Could you check a few things on this model? Use its own coordinates, in mm. A direction names the side the tool comes from. Give positions to 0.01 mm unless a question says otherwise; leave off trailing zeros. Order: outer loops, then holes, each group sorted by start corner. A loop starts at its lowest first (then second) coordinate and runs counter-clockwise, first axis right, second up. Notation, with made-up numbers: M -40,-39 L -16,-39 A35 cw -16,-5 Z; hole C 19,40.25 d8. An arc over 180 degrees is marked long. Use a Markdown table: item, result. Add a question column.
Autodesk Inventor part; units mm, degrees
ref_plane "YZ Plane" through (0, 0, 0) normal (1, 0, 0) x (0, 1, 0)
ref_plane "XZ Plane" through (0, 0, 0) normal (0, 1, 0) x (-1, 0, 0)
ref_plane "XY Plane" through (0, 0, 0) normal (0, 0, 1) x (1, 0, 0)
sketch "Skizze1" plane through (0, 0, 0) normal (0, 0, 1) x (1, 0, 0)
  line L0 (-21, 21) -> (21, 21)
  line L1 (21, 21) -> (21, -21)
  line L2 (21, -21) -> (-21, -21)
  line L3 (-21, -21) -> (-21, 21)
  line L4 (-29.4, 0) -> (29.4, 0)
  line L5 (0, -29.4) -> (0, 29.4)
  point P0 (0, 0)
  dimension "d0" = 42
  dimension "d1" = 42
extrude "Extrusion1" add sketch "Skizze1" along normal blind 50
sketch "Skizze2" plane through (0, 0, 50) normal (0, 0, 1) x (1, 0, 0)
  circle A0 centre (0, 0) radius 11
  dimension "d4" = 22
extrude "Extrusion2" add sketch "Skizze2" along normal blind 2
sketch "Skizze3" plane through (0, 0, 52) normal (0, 0, 1) x (1, 0, 0)
  circle A0 centre (0, 0) radius 11
  circle A1 centre (0, 0) radius 2.5
  dimension "d7" = 5
extrude "Extrusion3" add sketch "Skizze3" along normal blind 22 contours A1
chamfer "Fase1" distance 5 angle 45 4 edges at (-21, -21, 25) (21, -21, 25) (21, 21, 25) (-21, 21, 25)
sketch "Skizze4" plane through (0, 0, 50) normal (0, 0, 1) x (1, 0, 0)
  line L0 (-15.5, 15.5) -> (15.5, 15.5)
  line L1 (15.5, 15.5) -> (15.5, -15.5)
  line L2 (15.5, -15.5) -> (-15.5, -15.5)
  line L3 (-15.5, -15.5) -> (-15.5, 15.5)
  line L4 (-29.4, 0) -> (29.4, 0)
  line L5 (0, -29.4) -> (0, 29.4)
  dimension "d13" = 31
hole "Bohrung1" at (-15.5, 15.5, 50) at (15.5, 15.5, 50) at (15.5, -15.5, 50) at (-15.5, -15.5, 50) direction (0, 0, -1) diameter 2.459 depth 4.5 tip angle 118
properties part number "Motor"
1) Suppose I cut it at A-A on z = 5. Please give me the cut outline in (x, y).
2) For faces 4 (the face through (21, 0, 25)), 5 (the face through (-0.54, 2.44, 62.85)), which set-ups out of +Z, -Z, +X, -X, +Y, -Y let a thin tool reach every point of the face, with its end or its side?
3) For pin 1 (1.5 mm diameter, centred on x = 15.5, y = 15.5, fed in from +Z); pin 2 (4 mm diameter, centred on x = 7, z = 53, fed in from +Y); pin 3 (12.5 mm diameter, centred on x = 8.5, y = 4.5, fed in from +Z), each with a flat end and sliding along its axis, tell me the tip position at first contact or that it passes through.
4) Suppose I cut it at B-B on y = 0. Please give me the cut outline in (x, z), and give its area (3 significant figures).
5) We'd pull the mould along Y, two halves only. Please class faces 1 (the face through (0, 0, 74)), 2 (the face through (-18, -19, 25)), 3 (the face through (-15.869, -16.673, 47.718)): pulls with the +Y half, pulls with the -Y half, needs draft (parallel to the pull), parting line crosses it, or undercut.
6) Suppose I cut it at D-D on y = 18. Please give me the cut outline in (x, z).
7) Please list where these lines run through material, in increasing order: line 1 (X direction, y = 15.5, z = 49.1); line 2 (X direction, y = -15, z = 47). Write a range as from..to.
Values found:
| question | item | result |
|---|---|---|
| 1 | outline | M -21,-16 L -16,-21 L 16,-21 L 21,-16 L 21,16 L 16,21 L -16,21 L -21,16 Z |
| 2 | face 4 | +Z, -Z, +X, +Y, -Y |
| 2 | face 5 | +Z |
| 3 | pin 1 | stops at z = 45.21 |
| 3 | pin 2 | stops at y = 9.66 |
| 3 | pin 3 | stops at z = 52 |
| 4 | outline | M -21,0 L 21,0 L 21,50 L 11,50 L 11,52 L 2.5,52 L 2.5,74 L -2.5,74 L -2.5,52 L -11,52 L -11,50 L -21,50 Z |
| 4 | area | 2,250 mm^2 |
| 5 | face 1 | needs draft |
| 5 | face 2 | pulls with the -Y half |
| 5 | face 3 | undercut |
| 6 | outline | M -19,0 L 19,0 L 19,50 L -19,50 Z |
| 7 | line 1 | x = -21..-16.73, -14.27..14.27, 16.73..21 |
| 7 | line 2 | x = -21..-16.62, -14.38..14.38, 16.62..21 |
